Geometry: final body of the model. Coordinates: model frame, mm. A direction names the side the tool comes from. Give positions to 0.01 mm unless a question says otherwise; leave off trailing zeros. Write each loop counter-clockwise with the first axis right and the second up, starting at its lowest first coordinate (ties: lowest second). Pieces come first, ordered by that corner, then holes. Notation, with made-up numbers: (83.5, 60) -> (109.5, 60) arc R20 cw to (109.5, 80) -> close; hole circle Ø10 at (0.5, 86.5). An arc over 180 degrees is marked (long way). Answer in a Markdown table with one row per item. Add a question column.
Item 1: Section query D-D on z = 0.5. Output: boundary loops of the cut face in (x, y).
Item 2: First-contact query: P1, Ø1.5, axis at x = -10, z = 5, coming from the +Y side; P2, Ø3, axis at x = -3.5, z = 7, coming from the -Y side. Flat tips, straight axial feed; report the tip coordinate or a pass-through.
Item 3: Section query C-C on z = 4.25. Output: boundary loops of the cut face in (x, y), plus the area to 3 significant figures.
Item 4: Section query A-A on x = -10. Output: boundary loops of the cut face in (y, z).
Item 5: Material intervals for probe 1 along X at (y, z) = (1.15, 5); probe 2 along X at (y, z) = (16.5, 5); probe 3 along Y at (x, z) = (-9, 2), sorted ascending. Write a range as from..to.
Item 6: Access query for faces 4 (the flat face through (-15.5, 31, 5)), 5 (the flat face through (-1, 25, 0)), 6 (the cylindrical face through (14.6, 3.86, 4.93)). Directions: +Z, -Z, +X, -X, +Y, -Y. A direction counts if a zero-diameter tool reaches every point of the face in a straight line with its end or side. Return the directions, or none.
Item 7: Draft query along X for faces 1 (the flat face through (17, 35, 5)), 2 (the flat face through (18.5, 18, 5)), 3 (the cylindrical face through (9.01, 1.52, 5.76)). Return one class per face: +X half, -X half, draft (parallel to the pull), parting line (faces both ways), or undercut.
Item 8: Section query B-B on y = 12.5. Output: boundary loops of the cut face in (x, z), plus the area to 3 significant figures.
```python
from build123d import *

# Parameters (mm, degrees)
BOSS_EXTRUDE1_DEPTH = 10
SKETCH2_R           = 1.25
CUT_EXTRUDE1_DEPTH  = 4


with BuildPart() as part:
    # Sketch1 → Boss-Extrude1 (new body)
    with BuildSketch(Plane.XY):
        with BuildLine():
            Line((-15.5, 27), (15.5, 27))
            Line((15.5, 27), (15.5, 35))
            Line((15.5, 35), (18.5, 35))
            Line((18.5, 35), (18.5, 0))
            Line((18.5, 0), (7.5, 0))
            Line((7.5, 0), (7.5, 3))
            Line((7.5, 3), (12.5, 3))
            ThreePointArc((12.5, 3), (14.621320344, 3.878679656), (15.5, 6))
            Line((15.5, 6), (15.5, 21))
            ThreePointArc((15.5, 21), (14.621320344, 23.121320344), (12.5, 24))
            Line((12.5, 24), (-12.5, 24))
            ThreePointArc((-12.5, 24), (-14.621320344, 23.121320344), (-15.5, 21))
            Line((-15.5, 21), (-15.5, 6))
            ThreePointArc((-15.5, 6), (-14.621320344, 3.878679656), (-12.5, 3))
            Line((-12.5, 3), (-7.5, 3))
            Line((-7.5, 3), (-7.5, 0))
            Line((-7.5, 0), (-18.5, 0))
            Line((-18.5, 0), (-18.5, 35))
            Line((-18.5, 35), (-15.5, 35))
            Line((-15.5, 35), (-15.5, 27))
        make_face()
    extrude(amount=BOSS_EXTRUDE1_DEPTH)

    # Sketch2 → Cut-Extrude1 (cut, through all)
    with BuildSketch(Plane(origin=(0, 3, 0), x_dir=(1, 0, 0), z_dir=(0, 1, 0))):
        with Locations((-10, -5)):
            Circle(SKETCH2_R)
        with Locations((10, -5)):
            Circle(SKETCH2_R)
    extrude(amount=-CUT_EXTRUDE1_DEPTH, mode=Mode.SUBTRACT)


solid = part.part
```
Findings below:
| question | item | result |
|---|---|---|
| 1 | outline | (-18.5, 0) -> (-7.5, 0) -> (-7.5, 3) -> (-12.5, 3) arc R3 cw to (-15.5, 6) -> (-15.5, 21) arc R3 cw to (-12.5, 24) -> (12.5, 24) arc R3 cw to (15.5, 21) -> (15.5, 6) arc R3 cw to (12.5, 3) -> (7.5, 3) -> (7.5, 0) -> (18.5, 0) -> (18.5, 35) -> (15.5, 35) -> (15.5, 27) -> (-15.5, 27) -> (-15.5, 35) -> (-18.5, 35) -> close |
| 2 | P1 | stops at y = 27 |
| 2 | P2 | stops at y = 24 |
| 3 | outline | (-18.5, 0) -> (-11, 0) -> (-11, 3) -> (-12.5, 3) arc R3 cw to (-15.5, 6) -> (-15.5, 21) arc R3 cw to (-12.5, 24) -> (12.5, 24) arc R3 cw to (15.5, 21) -> (15.5, 6) arc R3 cw to (12.5, 3) -> (11, 3) -> (11, 0) -> (18.5, 0) -> (18.5, 35) -> (15.5, 35) -> (15.5, 27) -> (-15.5, 27) -> (-15.5, 35) -> (-18.5, 35) -> close; (-9, 0) -> (-7.5, 0) -> (-7.5, 3) -> (-9, 3) -> close; (7.5, 0) -> (9, 0) -> (9, 3) -> (7.5, 3) -> close |
| 3 | area | 347 mm^2 |
| 4 | outline | (0, 0) -> (3, 0) -> (3, 3.75) -> (0, 3.75) -> close; (0, 6.25) -> (3, 6.25) -> (3, 10) -> (0, 10) -> close; (24, 0) -> (27, 0) -> (27, 10) -> (24, 10) -> close |
| 5 | probe 1 | x = -18.5..-11.25, -8.75..-7.5, 7.5..8.75, 11.25..18.5 |
| 5 | probe 2 | x = -18.5..-15.5, 15.5..18.5 |
| 5 | probe 3 | y = 0..3, 24..27 |
| 6 | face 4 | +Z, -Z, +Y |
| 6 | face 5 | -Z, +X, -X, +Y, -Y |
| 6 | face 6 | +Z, -Z |
| 7 | face 1 | draft |
| 7 | face 2 | +X half |
| 7 | face 3 | undercut |
| 8 | outline | (-18.5, 0) -> (-15.5, 0) -> (-15.5, 10) -> (-18.5, 10) -> close; (15.5, 0) -> (18.5, 0) -> (18.5, 10) -> (15.5, 10) -> close |
| 8 | area | 60.0 mm^2 |
